from build123d import *

# Parameters (mm, degrees)
SKETCH1_R           = 3.2500000000000004
BOSS_EXTRUDE1_DEPTH = 3.5
SKETCH5_W           = 3.0499999999999994
SKETCH5_H           = 2.603568585765487
SKETCH7_R           = 2.5500000000000003
CUT_EXTRUDE1_DEPTH  = 1.8
SKETCH8_R           = 1.05
CUT_EXTRUDE2_DEPTH  = 12.484881366397794
FILLET1_R           = 1


with BuildPart() as part:
    # Sketch1 → Boss-Extrude1 (new body)
    with BuildSketch(Plane(origin=(0, 0, 0), x_dir=(1, 0, 0), z_dir=(0, 1, 0))):
        with Locations(Location((0, 0, 0), (0, 0, 270))):
            Circle(SKETCH1_R)
    extrude(amount=BOSS_EXTRUDE1_DEPTH)

    # Sweep2: read off the stored shape, not the designer's step
    # Sweep2 outline → Sweep2 (revolve)
    with BuildSketch(Plane.XY):
        with BuildLine():
            Line((0, 12.5), (0, 3.499999997))
            Line((0, 3.499999997), (2.999999996, 3.499999997))
            ThreePointArc((2.999999996, 3.499999997), (4.743416491, 9.081138828), (0, 12.5))
        make_face()
    revolve(axis=Axis((0, 0, 0), (0, 1, 0)))

    # Cut-Sweep2: sweep along a curve in space
    with BuildLine() as cut_sweep2_path:
        ThreePointArc((0, 3.4999999999999996, 3.000000000000002), (2.121320343559644, 3.4999999999999996, 2.121320343559644), (3.000000000000002, 3.4999999999999996, 0))
        ThreePointArc((3.000000000000002, 3.4999999999999996, 0), (2.121320343559644, 3.4999999999999996, -2.121320343559644), (0, 3.4999999999999996, -3.000000000000002))
        ThreePointArc((0, 3.4999999999999996, -3.000000000000002), (-2.121320343559644, 3.4999999999999996, -2.121320343559644), (-3.000000000000002, 3.4999999999999996, 0))
        ThreePointArc((-3.000000000000002, 3.4999999999999996, 0), (-2.121320343559644, 3.4999999999999996, 2.121320343559644), (0, 3.4999999999999996, 3.000000000000002))
    # Sketch5 → Cut-Sweep2 (sweep, cut)
    with BuildSketch(Plane.XY):
        with Locations((1.5249999999999997, 12.151784292882743)):
            Rectangle(SKETCH5_W, SKETCH5_H)
    sweep(path=cut_sweep2_path.line, mode=Mode.SUBTRACT)

    # Sketch7 → Cut-Extrude1 (cut)
    with BuildSketch(Plane(origin=(0, 10.85, 0), x_dir=(1, 0, 0), z_dir=(0, 1, 0))):
        with Locations(Location((0, 0, 0), (0, 0, 270))):
            Circle(SKETCH7_R)
    extrude(amount=-CUT_EXTRUDE1_DEPTH, mode=Mode.SUBTRACT)

    # Sketch8 → Cut-Extrude2 (cut, through all)
    with BuildSketch(Plane(origin=(0, 9.05, 0), x_dir=(1, 0, 0), z_dir=(0, 1, 0))):
        with Locations(Location((0, 0, 0), (0, 0, 270))):
            Circle(SKETCH8_R)
    extrude(amount=-CUT_EXTRUDE2_DEPTH, mode=Mode.SUBTRACT)

    # Fillet1
    # the kernel refuses this fillet: 1 mm, written as the material it adds along each edge
    with BuildSketch(Plane(origin=(0, 3.4999999970000006, 0), x_dir=(1, 0, 0), z_dir=(0, 0, 1))) as fillet1_piece_1:
        with BuildLine():
            CenterArc((4.21199518408407, -0.27306640979926655), FILLET1_R, 134.58762076250994, 29.565561163496568)
            ThreePointArc((3.5099959867224584, 0.4391113256738759), (3.2623943067411867, 0.21096537839129237), (2.9999999959999997, 0))
            Line((2.9999999959999997, 0), (3.250000000000001, 2.99999936e-09))
        make_face()
    revolve(axis=Axis((0, 3.4999999970000006, 0), (0, 1, 0)))


solid = part.part
Model file for the job. Use its own axes, mm. A direction names the side the tool comes from. Give positions to 0.01 mm unless a question says otherwise; leave off trailing zeros. Order: outer loops, then holes, each group sorted by start corner. A loop starts at its lowest first (then second) coordinate and runs counter-clockwise, first axis right, second up. Notation, with made-up numbers: M 27,72 L 49,72 A15 ccw 49,84 Z; hole C 11,4 d8. An arc over 180 degrees is marked long. Put each result on its own line as item: value. Start each with the question number.
(1) Band-saw the part on B-B on x = -4. Give the cut face in (y, z), then the cut area to 3 significant figures.
(2) Pin check, flat tips, straight feed: pin 1 Ø3 at (x, y) = (3, 2) entering from +Z; pin 2 Ø3.5 at (x, z) = (0, 0) entering from -Y; pin 3 Ø1.5 at (x, z) = (-2.5, 3) entering from +Y; pin 4 Ø1.7 at (x, z) = (0, 0) entering from -Y. Stop position of each tip, or through.
(3) Tool access for faces 1 (the face through (3.222, 1.726, -0.423)), 2 (the face through (1, 0, -1)), 3 (the face through (0.77, 9.96, 2.43)): list every direction of +Z, -Z, +X, -X, +Y, -Y with a clear straight run to the whole face (end or side of a thin tool).
(4) Drill centre lines: L1, parallel to X at y = 2.5, z = 0; L2, parallel to Z at x = 0, y = 11.3; L3, parallel to Y at x = 0.25, z = -2. Where is each one in solid material? Low to high. Write a range as [from, to].
(5) Band-saw the part on A-A on y = 10.5. Give the cut face in (x, z).
(6) Band-saw the part on C-C on y = 5.75. Give the cut face in (x, z), then the cut area to 3 significant figures.
Results below:
1. outline: C 7.5,0 d6
1. area: 28.3 mm2
2. pin 1: stops at z = 2.88
2. pin 2: stops at y = 0
2. pin 3: stops at y = 11.38
2. pin 4: passes through
3. face 1: -Y
3. face 2: +Z, -Z, +X, -X, -Y
3. face 3: +Y
4. L1: x = [-3.25, -1.05], [1.05, 3.25]
4. L2: z = [-3.25, -3.05], [3.05, 3.25]
4. L3: y = [0, 9.05]
5. outline: C 0,0 d8; hole C 0,0 d5.1
6. outline: C 0,0 d9.37; hole C 0,0 d2.1
6. area: 65.5 mm2
